from build123d import *

# Parameters (mm, degrees)
F0_W     = 6.217202
F0_H     = 6.892985
F0_H_2   = 6.926774
F0_W_2   = 5.338685
F0_H_3   = 6.28478
F0_W_3   = 6.217203
F0_W_4   = 1.721302
F0_H_4   = 3.012278
F0_W_5   = 1.721301
F1_DEPTH = 5.842
F2_DEPTH = 3.175


with BuildPart() as f1:
    # F0 (on Top) → F1 (new body)
    with BuildSketch(Plane.XY):
        with BuildLine():
            ThreePointArc((-3.276264, 19.408396), (-4.734943, 18.662064), (-6.193622, 19.408396))
            Line((-6.193622, 19.408396), (-7.051337, 19.263395))
            ThreePointArc((-7.051337, 19.263395), (-4.734943, 17.844209), (-2.41855, 19.263395))
            Line((-2.41855, 19.263395), (-3.276264, 19.408396))
        make_face()
        with BuildLine():
            ThreePointArc((-2.41855, 19.263395), (-4.734943, 17.844209), (-7.051337, 19.263395))
            Line((-7.051337, 19.263395), (-14.532115, 17.998736))
            Line((-14.532115, 17.998736), (-14.532115, 16.612969))
            Line((-14.532115, 16.612969), (-15.296676, 16.612969))
            Line((-15.296676, 16.612969), (-15.296676, 15.227202))
            Line((-15.296676, 15.227202), (-16.085131, 15.227202))
            Line((-16.085131, 15.227202), (-16.085131, 12.288421))
            Line((-16.085131, 12.288421), (-15.296676, 12.288421))
            Line((-15.296676, 12.288421), (-15.296676, -19.651944))
            Line((-15.296676, -19.651944), (-16.13486, -20.17758))
            Line((-16.13486, -20.17758), (-16.13486, -21.491669))
            Line((-16.13486, -21.491669), (-4.734943, -21.491669))
            Line((-4.734943, -21.491669), (6.664974, -21.491669))
            Line((6.664974, -21.491669), (6.664974, -20.17758))
            Line((6.664974, -20.17758), (5.82679, -19.651944))
            Line((5.82679, -19.651944), (5.82679, 12.288421))
            Line((5.82679, 12.288421), (6.615245, 12.288421))
            Line((6.615245, 12.288421), (6.615245, 15.227202))
            Line((6.615245, 15.227202), (5.82679, 15.227202))
            Line((5.82679, 15.227202), (5.82679, 16.612969))
            Line((5.82679, 16.612969), (5.062229, 16.612969))
            Line((5.062229, 16.612969), (5.062229, 17.998736))
            Line((5.062229, 17.998736), (-2.41855, 19.263395))
        make_face()
        with Locations((-10.101553, -15.893294)):
            Rectangle(F0_W, F0_H, mode=Mode.SUBTRACT)
        with Locations((-10.101553, -7.63185)):
            Rectangle(F0_W, F0_H_2, mode=Mode.SUBTRACT)
        with Locations((-10.101553, 0.494439)):
            Rectangle(F0_W_2, F0_H_3, mode=Mode.SUBTRACT)
        with Locations((0.631666, -15.893294)):
            Rectangle(F0_W_3, F0_H, mode=Mode.SUBTRACT)
        with Locations((0.631666, -7.63185)):
            Rectangle(F0_W_3, F0_H_2, mode=Mode.SUBTRACT)
        Polygon((-5.378293, 11.577819), (-4.734943, 11.577819), (-4.091593, 11.577819), (-4.091593, -19.293765), (-4.734943, -19.293765), (-5.378293, -19.293765), align=None, mode=Mode.SUBTRACT)
        with Locations((0.631666, 0.494439)):
            Rectangle(F0_W_2, F0_H_3, mode=Mode.SUBTRACT)
        with Locations((-12.23792, 6.726886)):
            Rectangle(F0_W_4, F0_H_4, mode=Mode.SUBTRACT)
        with Locations((-12.23792, 10.126886)):
            Rectangle(F0_W_4, F0_H_4, mode=Mode.SUBTRACT)
        with Locations((-10.08792, 6.726886)):
            Rectangle(F0_W_4, F0_H_4, mode=Mode.SUBTRACT)
        with Locations((-7.93792, 6.726886)):
            Rectangle(F0_W_4, F0_H_4, mode=Mode.SUBTRACT)
        with Locations((-10.08792, 10.126886)):
            Rectangle(F0_W_4, F0_H_4, mode=Mode.SUBTRACT)
        with Locations((-7.93792, 10.126886)):
            Rectangle(F0_W_4, F0_H_4, mode=Mode.SUBTRACT)
        with Locations((-1.531967, 6.726886)):
            Rectangle(F0_W_5, F0_H_4, mode=Mode.SUBTRACT)
        with Locations((0.618033, 6.726886)):
            Rectangle(F0_W_5, F0_H_4, mode=Mode.SUBTRACT)
        with Locations((-1.531967, 10.126886)):
            Rectangle(F0_W_5, F0_H_4, mode=Mode.SUBTRACT)
        with Locations((0.618033, 10.126886)):
            Rectangle(F0_W_5, F0_H_4, mode=Mode.SUBTRACT)
        with Locations((2.768033, 6.726886)):
            Rectangle(F0_W_5, F0_H_4, mode=Mode.SUBTRACT)
        with Locations((2.768033, 10.126886)):
            Rectangle(F0_W_5, F0_H_4, mode=Mode.SUBTRACT)
        Polygon((-14.532275, 14.731877), (-4.734943, 14.731877), (5.062388, 14.731877), (5.062388, 12.823218), (-4.734943, 12.823218), (-14.532275, 12.823218), align=None, mode=Mode.SUBTRACT)
    extrude(amount=F1_DEPTH)

    # F0 (on Top) → F2 (join)
    with BuildSketch(Plane.XY):
        with BuildLine():
            Line((-5.667986, 21.749863), (-4.734943, 22.132145))
            Line((-4.734943, 22.132145), (-3.8019, 21.749863))
            Line((-3.8019, 21.749863), (-3.8019, 20.053495))
            Line((-3.8019, 20.053495), (-3.276264, 20.053495))
            Line((-3.276264, 20.053495), (-3.276264, 19.408396))
            Line((-3.276264, 19.408396), (-2.41855, 19.263395))
            ThreePointArc((-2.41855, 19.263395), (-2.206839, 19.837012), (-2.134943, 20.444209))
            ThreePointArc((-2.134943, 20.444209), (-5.34214, 22.972313), (-7.051337, 19.263395))
            Line((-7.051337, 19.263395), (-6.193622, 19.408396))
            Line((-6.193622, 19.408396), (-6.193622, 20.053495))
            Line((-6.193622, 20.053495), (-5.667986, 20.053495))
            Line((-5.667986, 20.053495), (-5.667986, 21.749863))
        make_face()
    extrude(amount=F2_DEPTH)


solid = f1.part
Could you check a few things on this model? Use its own coordinates, in mm. A direction names the side the tool comes from. Coordinates: 2 decimals unless noted, no trailing zeros. Order: outer loops, then holes, each group sorted by start corner. A loop starts at its lowest first (then second) coordinate and runs counter-clockwise, first axis right, second up. Notation, with made-up numbers: (85.25, 46) - (132.25, 46) arc R31 cw to (132.25, 78) - close; hole circle Ø3 at (53.5, -9.5). An arc over 180 degrees is marked (long way). Answer in a Markdown table with one row per item. Add a question column.
(1) I need wall thicknesses on L1, parallel to X at y = -9.5, z = 3.35; L2, parallel to X at y = 0, z = 3.15; L3, parallel to Y at x = -3.5, z = 2.1. Which ranges of each line are inside material? Lowest first, please.
(2) If we section it at C-C, the plane z = 0.75: State how many separate pieces and enclosed holes the cut face has, then the cut area to 3 significant figures.
(3) If we section it at A-A, the plane y = -7: Please give me the cut outline in (x, z), then the cut area to 3 significant figures.
(4) If we section it at B-B, the plane x = -10.5: Please give me the cut outline in (y, z), then the cut area to 3 significant figures.
(5) Will these pins go through, and if not, where does the flat tip stop? pin 1 (0.9 mm diameter, centred on x = -2, z = 2, fed in from +Y); pin 2 (0.9 mm diameter, centred on y = 10, z = 2, fed in from -X); pin 3 (3 mm diameter, centred on y = -14.5, z = 3.5, fed in from +X); pin 4 (2 mm diameter, centred on x = 2, y = 8, fed in from -Z).
(6) On a 3-axis mill with a long thin cutter (end or side, diameter ignored), from which of +Z, -Z, +X, -X, +Y, -Y can I reach the whole of each face in a straight line? I mean faces 1 (the face through (5.827, -4, 3)), 2 (the face through (-10, -4.168, 3)), 3 (the face through (-2.4, 1.1, 0)). Say none if no direction works.
(7) If we mould it in two halves opening along X, with no side actions, what happens to faces 4 (the face through (-16.135, -21, 3)), 5 (the face through (-6.993, -16, 3)), 6 (the face through (6.615, 14, 3))? For each: released by +X, released by -X, zero draft, split by the parting line, or undercut.
Results are:
| question | item | result |
|---|---|---|
| 1 | L1 | x = -15.3 to -13.21, -6.99 to -5.38, -4.09 to -2.48, 3.74 to 5.83 |
| 1 | L2 | x = -15.3 to -12.77, -7.43 to -5.38, -4.09 to -2.04, 3.3 to 5.83 |
| 1 | L3 | y = -21.49 to 12.82, 14.73 to 19.15, 20.05 to 22.73 |
| 2 | separate pieces | 1 |
| 2 | enclosed holes | 21 |
| 2 | area | 486 mm2 |
| 3 | outline | (-15.3, 0) - (-13.21, 0) - (-13.21, 5.84) - (-15.3, 5.84) - close; (-6.99, 0) - (-5.38, 0) - (-5.38, 5.84) - (-6.99, 5.84) - close; (-4.09, 0) - (-2.48, 0) - (-2.48, 5.84) - (-4.09, 5.84) - close; (3.74, 0) - (5.83, 0) - (5.83, 5.84) - (3.74, 5.84) - close |
| 3 | area | 43.2 mm2 |
| 4 | outline | (-21.49, 0) - (-19.34, 0) - (-19.34, 5.84) - (-21.49, 5.84) - close; (-12.45, 0) - (-11.1, 0) - (-11.1, 5.84) - (-12.45, 5.84) - close; (-4.17, 0) - (-2.65, 0) - (-2.65, 5.84) - (-4.17, 5.84) - close; (3.64, 0) - (5.22, 0) - (5.22, 5.84) - (3.64, 5.84) - close; (8.23, 0) - (8.62, 0) - (8.62, 5.84) - (8.23, 5.84) - close; (11.63, 0) - (12.82, 0) - (12.82, 5.84) - (11.63, 5.84) - close; (14.73, 0) - (18.68, 0) - (18.68, 5.84) - (14.73, 5.84) - close |
| 4 | area | 70.9 mm2 |
| 5 | pin 1 | stops at y = 21.68 |
| 5 | pin 2 | stops at x = -15.3 |
| 5 | pin 3 | stops at x = 5.83 |
| 5 | pin 4 | stops at z = 0 |
| 6 | face 1 | +Z, -Z, +X |
| 6 | face 2 | +Z, -Z |
| 6 | face 3 | -Z, +X, -X, +Y, -Y |
| 7 | face 4 | released by -X |
| 7 | face 5 | undercut |
| 7 | face 6 | released by +X |
